```python
from build123d import *

# Parameters (mm, degrees)
EXTRUDE_1_DEPTH     = 17.5
CUT_EXTRUDE_1_DEPTH = 14.5
CUT_EXTRUDE_2_REACH = 42
CUT_EXTRUDE_3_REACH = 42


with BuildPart() as part:
    # 草图1 → 凸台-拉伸1 (new body, symmetric)
    with BuildSketch(Plane.XY):
        Polygon((0, 40), (0, 0), (40, 0), (40, 8), (30, 8), (8, 30), (8, 40), align=None)
    extrude(amount=EXTRUDE_1_DEPTH, both=True)

    # 草图2 → 切除-拉伸1 (cut, symmetric)
    with BuildSketch(Plane.XY):
        Polygon((4.5, 40), (4.5, 4.5), (40, 4.5), (40, 8), (8, 40), align=None)
    extrude(amount=CUT_EXTRUDE_1_DEPTH, both=True, mode=Mode.SUBTRACT)

    # 草图3 → 切除-拉伸2 (cut, up to next)
    with BuildSketch(Plane.XZ, mode=Mode.PRIVATE) as cut_extrude_2_sk1:
        with BuildLine():
            Line((13, -4.5), (27, -4.5))
            ThreePointArc((27, -4.5), (31.5, 0), (27, 4.5))
            Line((27, 4.5), (13, 4.5))
            ThreePointArc((13, 4.5), (8.5, 0), (13, -4.5))
        make_face()
    cut_extrude_2_tool1 = extrude(cut_extrude_2_sk1.sketch, amount=-CUT_EXTRUDE_2_REACH, mode=Mode.PRIVATE) & part.part
    add(cut_extrude_2_tool1.solids().sort_by_distance((20, 0, 0))[0], mode=Mode.SUBTRACT)

    # 草图4 → 切除-拉伸3 (cut, up to next)
    with BuildSketch(Plane.ZY, mode=Mode.PRIVATE) as cut_extrude_3_sk1:
        with BuildLine():
            Line((4.5, 15), (4.5, 30))
            ThreePointArc((4.5, 30), (0, 34.5), (-4.5, 30))
            Line((-4.5, 30), (-4.5, 15))
            ThreePointArc((-4.5, 15), (0, 10.5), (4.5, 15))
        make_face()
    cut_extrude_3_tool1 = extrude(cut_extrude_3_sk1.sketch, amount=-CUT_EXTRUDE_3_REACH, mode=Mode.PRIVATE) & part.part
    add(cut_extrude_3_tool1.solids().sort_by_distance((0, 22.5, 0))[0], mode=Mode.SUBTRACT)


solid = part.part
```
Could you check a few things on this model? Use its own coordinates, in mm. A direction names the side the tool comes from. Give positions to 0.01 mm unless a question says otherwise; leave off trailing zeros. Write each loop counter-clockwise with the first axis right and the second up, starting at its lowest first coordinate (ties: lowest second). Pieces come first, ordered by that corner, then holes. Notation, with made-up numbers: (-12.75, -14.75) -> (-6.75, -14.75) arc R30 ccw to (-6.75, 11.25) -> close; hole circle Ø11 at (66, -8). An arc over 180 degrees is marked (long way). Write each question's results on one line, items separated by ' | '.
1. Will these pins go through, and if not, where does the flat tip stop? pin 1 Ø2.5 at (x, z) = (35, 15.5) entering from +Y; pin 2 Ø1.5 at (y, z) = (30.5, -11.5) entering from +X; pin 3 Ø12 at (y, z) = (36, -10.5) entering from +X.
Check sheet entries:
pin 1: stops at y = 8 | pin 2: stops at x = 4.5 | pin 3: stops at x = 8
2. I want a section at C-C, the plane y = 14. Write out the boundary of the cut face in (x, z), then the cut area to 3 significant figures.
Check sheet entries:
outline: (0, -17.5) -> (24, -17.5) -> (24, -14.5) -> (4.5, -14.5) -> (4.5, -4.39) -> (0, -4.39) -> close; (0, 4.39) -> (4.5, 4.39) -> (4.5, 14.5) -> (24, 14.5) -> (24, 17.5) -> (0, 17.5) -> close | area: 235 mm²
3. I want a section at B-B, the plane z = 0. Write out the boundary of the cut face in (x, y).
Check sheet entries:
outline: (0, 0) -> (8.5, 0) -> (8.5, 4.5) -> (4.5, 4.5) -> (4.5, 10.5) -> (0, 10.5) -> close; (0, 34.5) -> (4.5, 34.5) -> (4.5, 40) -> (0, 40) -> close; (31.5, 0) -> (40, 0) -> (40, 4.5) -> (31.5, 4.5) -> close
4. I want a section at A-A, the plane x = 19.5. Write out the boundary of the cut face in (y, z), then the cut area to 3 significant figures.
Check sheet entries:
outline: (0, -17.5) -> (18.5, -17.5) -> (18.5, -14.5) -> (4.5, -14.5) -> (4.5, -4.5) -> (0, -4.5) -> close; (0, 4.5) -> (4.5, 4.5) -> (4.5, 14.5) -> (18.5, 14.5) -> (18.5, 17.5) -> (0, 17.5) -> close | area: 201 mm²
5. If we mould it in two halves opening along Z, with no side actions, what happens to faces 6 (the flat face through (35, 8, 16)), 7 (the flat face through (2, 22, 4.5)), 8 (the flat face through (14, 15, -14.5)), 9 (the flat face through (15, 16, -17.5))? For each: released by +Z, released by -Z, zero draft, split by the parting line, or undercut.
Check sheet entries:
face 6: zero draft | face 7: undercut | face 8: undercut | face 9: released by -Z
6. I need wall thicknesses on L1, parallel to Z at x = 6.5, y = 5.5; L2, parallel to Z at x = 2, y = 21.5; L3, parallel to X at y = 31.5, z = -12. Which ranges of each line are inside material? Lowest first, please.
Check sheet entries:
L1: z = -17.5 to -14.5, 14.5 to 17.5 | L2: z = -17.5 to -4.5, 4.5 to 17.5 | L3: x = 0 to 4.5
7. I want a section at D-D, the plane z = 7. Write out the boundary of the cut face in (x, y).
Check sheet entries:
outline: (0, 0) -> (40, 0) -> (40, 4.5) -> (4.5, 4.5) -> (4.5, 40) -> (0, 40) -> close
8. On a 3-axis mill with a long thin cutter (end or side, diameter ignored), from which of +Z, -Z, +X, -X, +Y, -Y can I reach the whole of each face in a straight line? I mean faces 1 (the flat face through (15, 16, 17.5)), 2 (the flat face through (8, 35, -16)), 3 (the flat face through (2, 23, -4.5)), 4 (the flat face through (22, 4.5, -6)), 5 (the cylindrical face through (31.5, 2.2, -0.1)). Say none if no direction works.
Check sheet entries:
face 1: +Z, +X, -X, +Y, -Y | face 2: +Z, -Z, +X, +Y | face 3: +X, -X | face 4: +X, +Y | face 5: +Y, -Y
